```python
from build123d import *

# Parameters (mm, degrees)
ESBO_O1_W                = 3.4999999999999996
ESBO_O1_H                = 2
RESSALTO_EXTRUS_O1_DEPTH = 5.5
CORTE_EXTRUS_O1_DEPTH    = 2.5
FILETE1_R                = 0.5
ESBO_O3_R                = 0.2500000000000004
ESBO_O3_R_2              = 0.25
RESSALTO_EXTRUS_O2_DEPTH = 16
ESBO_O4_R                = 0.35087883808626286
CORTE_EXTRUS_O2_DEPTH    = 3.9999999999999933


with BuildPart() as part:
    # Esboço1 → Ressalto-extrusão1 (new body)
    with BuildSketch(Plane.XY):
        with Locations((1.7499999999999998, -1)):
            Rectangle(ESBO_O1_W, ESBO_O1_H)
    extrude(amount=RESSALTO_EXTRUS_O1_DEPTH)

    # Esboço2 → Corte-extrusão1 (cut)
    with BuildSketch(Plane.XY.offset(5.5)):
        with BuildLine():
            Line((0, -2), (1.7499999999999791, -1.9999999999999998))
            ThreePointArc((1.7499999999999791, -2), (0.7499999999999996, -1.000000000000021), (1.7499999999999365, 2.2e-16))
            Line((1.7499999999999365, 0), (0, 0))
            Line((0, 0), (0, -2))
        make_face()
        with BuildLine():
            Line((1.7499999999999791, -1.9999999999999998), (3.4999999999999996, -1.9999999999999996))
            Line((3.4999999999999996, -1.9999999999999996), (3.4999999999999996, 0))
            Line((3.4999999999999996, 0), (1.7499999999999365, 0))
            ThreePointArc((1.7499999999999365, 2.2e-16), (2.457106781186525, -0.29289321881343), (2.75, -1))
            ThreePointArc((2.75, -1.0000000000000002), (2.4571067811865404, -1.7071067811865546), (1.7499999999999791, -2))
        make_face()
    extrude(amount=-CORTE_EXTRUS_O1_DEPTH, mode=Mode.SUBTRACT)

    # Filete1
    filete1_edges = [part.edges().sort_by_distance(p)[0] for p in [
        (1.7500000000000198, 2.2e-16, 5.5),
    ]]
    fillet(filete1_edges, radius=FILETE1_R)

    # Esboço3 → Ressalto-extrusão2 (add)
    with BuildSketch(Plane(origin=(0, 0, 0), x_dir=(-1, 0, 0), z_dir=(0, 0, -1))):
        with Locations(Location((-3.05, -1, 0), (0, 0, 180))):
            Circle(ESBO_O3_R)
        with Locations(Location((-0.45, -1, 0), (0, 0, 180))):
            Circle(ESBO_O3_R_2)
    extrude(amount=RESSALTO_EXTRUS_O2_DEPTH)

    # Esboço4 → Corte-extrusão2 (cut)
    with BuildSketch(Plane(origin=(0, 0, -16), x_dir=(-1, 0, 0), z_dir=(0, 0, -1))):
        with Locations((-0.45, -1)):
            Circle(ESBO_O4_R)
    extrude(amount=-CORTE_EXTRUS_O2_DEPTH, mode=Mode.SUBTRACT)


solid = part.part
```
Could you check a few things on this model? Use its own coordinates, in mm. A direction names the side the tool comes from. Round coordinates to 2 decimals unless told otherwise and drop trailing zeros. Loops run counter-clockwise (first coordinate to the right, second up) from the corner with the lowest first, then second, coordinate; pieces in that order, holes last. Notation, with made-up numbers: M 68.5,38.5 L 86.5,38.5 A10 ccw 86.5,54.5 Z; hole C -27.75,-7 d4. An arc over 180 degrees is marked long. Put each result on its own line as item: value.
Q1. Imagine slicing it at A-A (x = 0.45). Write out the boundary of the cut face in (y, z).
Check result:
outline: M -2,0 L -1.25,0 L -1.25,-12 L -0.75,-12 L -0.75,0 L 0,0 L 0,3 L -2,3 Z
Q2. Imagine slicing it at D-D (x = 3.05). Write out the boundary of the cut face in (y, z).
Check result:
outline: M -2,0 L -1.25,0 L -1.25,-16 L -0.75,-16 L -0.75,0 L 0,0 L 0,3 L -2,3 Z
Q3. For pin 1 (0.9 mm diameter, centred on x = 0.5, y = -1, fed in from +Z); pin 2 (0.5 mm diameter, centred on x = 0.5, y = -1, fed in from -Z); pin 3 (1 mm diameter, centred on x = 1.5, y = -1, fed in from -Z), each with a flat end and sliding along its axis, tell me the tip position at first contact or that it passes through.
Check result:
pin 1: z = 5.4
pin 2: z = -12
pin 3: z = 0
Q4. Imagine slicing it at C-C (z = -14.5). Write out the boundary of the cut face in (x, y), then the cut area to 3 significant figures.
Check result:
outline: C 3.05,-1 d0.5
area: 0.196 mm2
Q5. On a 3-axis mill with a long thin cutter (end or side, diameter ignored), from which of +Z, -Z, +X, -X, +Y, -Y can I reach the whole of each face in a straight line? I mean faces 1 (the face through (2, -1, 5.5)), 2 (the face through (2.726, -0.783, 4.014)). Say none if no direction works.
Check result:
face 1: +Z, +X, -X, +Y, -Y
face 2: +Z
Q6. Imagine slicing it at B-B (z = -8). Write out the boundary of the cut face in (x, y), then the cut area to 3 significant figures.
Check result:
outline: C 0.45,-1 d0.5; C 3.05,-1 d0.5
area: 0.393 mm2
Q7. I need wall thicknesses on probe 1 along Z at (x, y) = (1.1, -0.05); probe 2 along Z at (x, y) = (2.85, -0.95); probe 3 along X at (y, z) = (-0.85, -2). Which ranges of each line are inside material? Lowest first, please.
Check result:
probe 1: 0 to 3
probe 2: -16 to 3
probe 3: 0.25 to 0.65, 2.85 to 3.25
Q8. Thinking about a two-plate mould opening in X: for faces 3 (the face through (3, -1, 3)), 4 (the face through (2, -1, 0)), 5 (the face through (3.5, -1, 1)), 6 (the face through (0, -1, 1)), which applies, released by +X, released by -X, zero draft, split by the parting line, or undercut?
Check result:
face 3: zero draft
face 4: undercut
face 5: released by +X
face 6: released by -X
